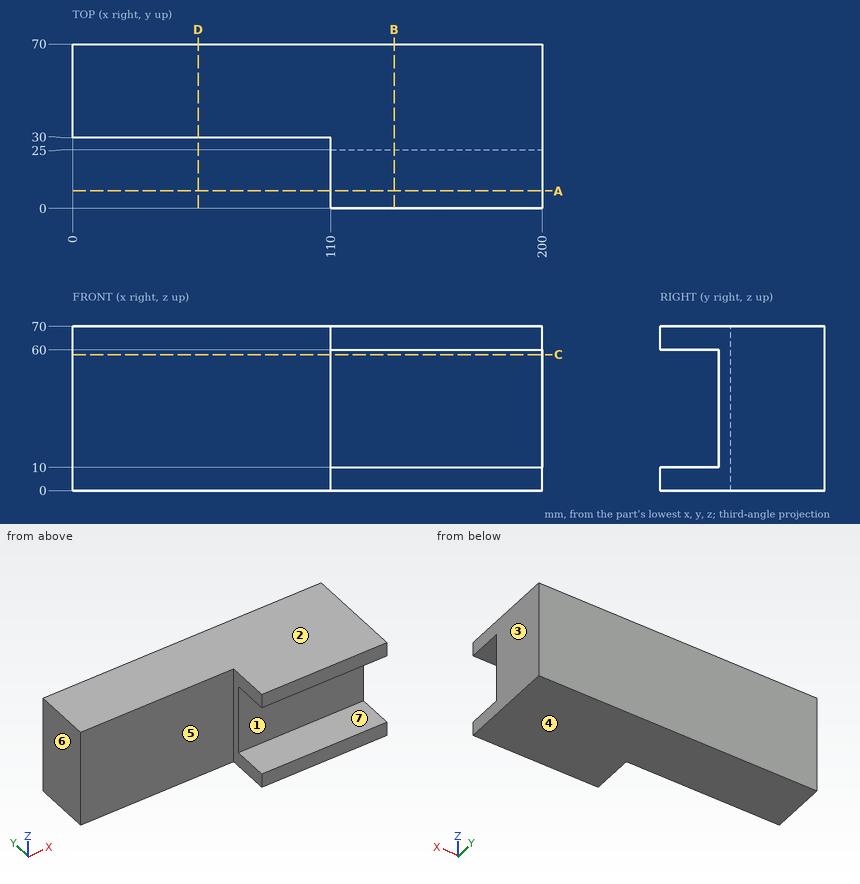
Could you check a few things on this drawing? It's one solid part, dimensions in mm from its lowest x, y, z. A direction names the side the tool comes from. Give positions to 0.01 mm unless a question says otherwise; leave off trailing zeros. Write each loop counter-clockwise with the first axis right and the second up, starting at its lowest first coordinate (ties: lowest second). Pieces come first, ordered by that corner, then holes. Notation, with made-up numbers: (55.5, -21.75) -> (61.5, -21.75) arc R8 ccw to (61.5, -13.75) -> close; hole circle Ø9 at (-28, 73). An arc over 180 degrees is marked (long way). Answer as a JSON object with one key per item and string values.
Q1. Suppose I cut it at A-A on y = 7.5. Write out the boundary of the cut face in (x, z), then the cut area to 3 significant figures.
Taken from the geometry:
{"outline": "(110, 0) -> (200, 0) -> (200, 10) -> (110, 10) -> close; (110, 60) -> (200, 60) -> (200, 70) -> (110, 70) -> close", "area": "1,800 mm²"}
Q2. Will these pins go through, and if not, where does the flat tip stop? pin 1 Ø1.5 at (x, z) = (32, 7) entering from -Y; pin 2 Ø8 at (x, z) = (114, 11.5) entering from -Y.
Taken from the geometry:
{"pin 1": "stops at y = 30", "pin 2": "stops at y = 0"}
Q3. Please list where these lines run through material, in increasing order: L1, parallel to Z at x = 171.5, y = 8.5; L2, parallel to Y at x = 145, z = 15; L3, parallel to Y at x = 42, z = 66.5.
Taken from the geometry:
{"L1": "z = 0 to 10, 60 to 70", "L2": "y = 25 to 70", "L3": "y = 30 to 70"}
Q4. Suppose I cut it at B-B on x = 137. Write out the boundary of the cut face in (y, z), then the cut area to 3 significant figures.
Taken from the geometry:
{"outline": "(0, 0) -> (70, 0) -> (70, 70) -> (0, 70) -> (0, 60) -> (25, 60) -> (25, 10) -> (0, 10) -> close", "area": "3,650 mm²"}
Q5. Suppose I cut it at D-D on x = 53.5. Write out the boundary of the cut face in (y, z).
Taken from the geometry:
{"outline": "(30, 0) -> (70, 0) -> (70, 70) -> (30, 70) -> close"}
Q6. We'd pull the mould along Z, two halves only. Please class the marked faces 1, 2, 3 and 4: released by +Z, released by -Z, zero draft, split by the parting line, or undercut.
Taken from the geometry:
{"face 1": "undercut", "face 2": "released by +Z", "face 3": "zero draft", "face 4": "released by -Z"}
Q7. Which directions (+Z, -Z, +X, -X, +Y, -Y) give clear straight access to the entire face, cutting with the end or side of a thin tool? Please do the marked faces 5, 6 and 7.
Taken from the geometry:
{"face 5": "+Z, -Z, -X, -Y", "face 6": "+Z, -Z, -X, +Y, -Y", "face 7": "+X, -X, -Y"}
Q8. Suppose I cut it at C-C on z = 58. Write out the boundary of the cut face in (x, y).
Taken from the geometry:
{"outline": "(0, 30) -> (110, 30) -> (110, 25) -> (200, 25) -> (200, 70) -> (0, 70) -> close"}
